Autodesk Inventor part; units mm, degrees
ref_plane "YZ Plane" through (0, 0, 0) normal (1, 0, 0) x (0, 1, 0)
ref_plane "XZ Plane" through (0, 0, 0) normal (0, 1, 0) x (-1, 0, 0)
ref_plane "XY Plane" through (0, 0, 0) normal (0, 0, 1) x (1, 0, 0)
sketch "Sketch1" plane through (0, 0, 0) normal (0, 1, 0) x (-1, 0, 0)
  line L0 (17, 250) -> (0, 250)
  line L1 (0, 250) -> (0, 0)
  line L2 (0, 0) -> (17, 0)
  line L3 (17, 0) -> (17, 250)
  line L4 (17, 0) -> (-233, 0)
  line L5 (-233, 0) -> (-233, -17)
  line L6 (-233, -17) -> (17, -17)
  line L7 (17, -17) -> (17, 0)
  dimension "d0" = 17
  dimension "d1" = 250
  dimension "d2" = 250
extrude "Extrusion1" add sketch "Sketch1" along normal blind 284.5
sketch "Sketch2" plane through (233, 0, -17) normal (0, 0, -1) x (-1, 0, 0)
  line L0 (0, 0) -> (250, 0)
  line L1 (250, 0) -> (250, 284.5)
  line L2 (0, 284.5) -> (250, 284.5)
  line L3 (0, 0) -> (0, 284.5)
  line L4 (182.1785, 237.4156) -> (168.1785, 237.4156)
  line L5 (168.1785, 237.4156) -> (168.1785, 159.4156)
  line L6 (168.1785, 159.4156) -> (182.1785, 159.4156)
  line L7 (182.1785, 159.4156) -> (182.1785, 237.4156)
  line L8 (168.1785, 208.4156) -> (82.1785, 208.4156)
  line L9 (82.1785, 208.4156) -> (82.1785, 188.4156)
  line L10 (82.1785, 188.4156) -> (168.1785, 188.4156)
  line L11 (168.1785, 188.4156) -> (168.1785, 208.4156)
  arc A0 (64.6656, 225.9286) -> (82.1785, 208.4156) centre (82.1785, 225.9286) ccw
  line L12 (82.1785, 225.9286) -> (64.6656, 225.9286) construction
  line L13 (82.1785, 225.9286) -> (82.1785, 208.4156) construction
  arc A1 (44.6656, 225.9286) -> (82.1785, 188.4156) centre (82.1785, 225.9286) ccw
  line L14 (64.6656, 225.9286) -> (44.6656, 225.9286)
  line L15 (182.3419, 116.525) -> (46.5005, 150.394)
  line L16 (46.5005, 150.394) -> (46.5005, 130.394)
  line L17 (46.5005, 130.394) -> (114.6042, 113.4139)
  line L18 (133.1096, 95.525) -> (133.1096, 103.525)
  line L19 (133.1096, 103.525) -> (163.0533, 95.5016)
  line L20 (114.6042, 113.4139) -> (114.6042, 93.4139)
  line L21 (182.3419, 116.525) -> (182.3419, 95.525)
  line L22 (133.1096, 95.525) -> (42.0362, 95.525)
  line L23 (182.3419, 74.525) -> (46.5005, 40.6559)
  line L24 (46.5005, 40.6559) -> (46.5005, 60.6559)
  line L25 (46.5005, 60.6559) -> (114.6042, 77.6361)
  line L26 (133.1096, 95.525) -> (133.1096, 87.525)
  line L27 (133.1096, 87.525) -> (163.0533, 95.5484)
  line L28 (114.6042, 77.6361) -> (114.6042, 97.6361)
  line L29 (182.3419, 74.525) -> (182.3419, 95.525)
  point P0 (233, 0)
  point P1 (162.966, 95.525)
  dimension "d5" = 90
  dimension "d6" = 21
  dimension "d7" = 140
  dimension "d8" = 20
  dimension "d9" = 20
  dimension "d10" = 8
  dimension "d11" = 31
  dimension "d12" = 68.1037
  dimension "d13" = 78
  dimension "d14" = 20
  dimension "d15" = 29
  dimension "d16" = 14
  dimension "d18" = 86
  dimension "d19" = 75
  dimension "d20" = 76
extrude "Extrusion2" cut sketch "Sketch2" against normal blind 1 contours L7 L6 L5 L4 | L5 L10 L9 L8 | L9 A1 L14 A0 | L21 L29 L23 L24 L25 L28 L20 L17 L16 L15
fillet "Fillet1" radius 3 19 edges at (50.6581, 116.525, -16.5) (99.8904, 87.525, -16.5) (99.8904, 103.525, -16.5) (70.034, 95.525, -16.5) (50.6581, 74.525, -16.5) (50.8215, 159.4156, -16.5) (64.8215, 188.4156, -16.5) (118.3958, 113.4139, -16.5) (118.3958, 77.6361, -16.5) (186.4995, 40.6559, -16.5) (186.4995, 60.6559, -16.5) (186.4995, 130.394, -16.5) (186.4995, 150.394, -16.5) (168.3344, 225.9286, -16.5) (188.3344, 225.9286, -16.5) (64.8215, 237.4156, -16.5) (50.8215, 237.4156, -16.5) (64.8215, 159.4156, -16.5) (64.8215, 208.4156, -16.5)
equation "\"d15\" = 0.5 * d13 - 0.5 * d14"
properties part number "TableroEscrito"
For this review, take the finished solid that the model builds, in its own axes (mm). A direction names the side the tool comes from. Coordinates: 2 decimals unless noted, no trailing zeros. Write each loop counter-clockwise with the first axis right and the second up, starting at its lowest first coordinate (ties: lowest second). Pieces come first, ordered by that corner, then holes. Notation, with made-up numbers: (85.25, -9) - (113.25, -9) arc R17 ccw to (113.25, 4) - close; hole circle Ø7 at (-24, 69.25). An arc over 180 degrees is marked (long way). Answer in a Markdown table with one row per item. Add a question column.
Q1. We need section A-A, the plane y = 30. State the section outline as (x, z) points, and give its area (3 significant figures).
Q2. For P1, Ø10, axis at y = 66.5, z = 157, coming from the +X side; P2, Ø1.5, axis at x = 81.5, y = 61.5, coming from the +Z side; P3, Ø0.5, axis at x = 123.5, z = -16.5, coming from the -Y side, all flat-tipped, find the tip position at first contact; note any pin that passes through.
Q3. Tool access review of faces 5 (the flat face through (116.94, 133.05, -16.51)), 6 (the flat face through (0, 140, 127)), 7 (the flat face through (-3, 0, 58)): name each direction out of +Z, -Z, +X, -X, +Y, -Y from which nothing blocks a thin tool from reaching the whole face with its end or side.
Q4. We need section B-B, the plane z = 227. State the section outline as (x, y) points, and give its area (3 significant figures).
Q5. Draft analysis for pull direction X (two halves, no side actions). For faces 1 (the flat face through (92, 95, -17)), 2 (the flat face through (105, 199, -16)), 3 (the flat face through (104, 96, -16)), 4 (the flat face through (233, 140, -8)), state which applies: +X half, -X half, draft (parallel to the pull), parting line (faces both ways), or undercut.
Q6. For probe 1 along Z at (x, y) = (188, 245); probe 2 along Z at (x, y) = (172, 208.5), list the stretches that pass through material, from the lowest coordinate up.
Q7. We need section C-C, the plane x = 199. State the section outline as (y, z) points.
Answer list:
| question | item | result |
|---|---|---|
| 1 | outline | (-17, -17) - (233, -17) - (233, 0) - (0, 0) - (0, 250) - (-17, 250) - close |
| 1 | area | 8,500 mm2 |
| 2 | P1 | stops at x = 0 |
| 2 | P2 | stops at z = 0 |
| 2 | P3 | stops at y = 0 |
| 3 | face 5 | -Z |
| 3 | face 6 | +Z, +X, +Y, -Y |
| 3 | face 7 | +Z, -Z, +X, -X, -Y |
| 4 | outline | (-17, 0) - (0, 0) - (0, 284.5) - (-17, 284.5) - close |
| 4 | area | 4,840 mm2 |
| 5 | face 1 | draft |
| 5 | face 2 | undercut |
| 5 | face 3 | undercut |
| 5 | face 4 | +X half |
| 6 | probe 1 | z = -17 to 0 |
| 6 | probe 2 | z = -16 to 0 |
| 7 | outline | (0, -17) - (284.5, -17) - (284.5, 0) - (0, 0) - close |
